Verification items for the finished model (mm, model axes). Face numbers are marked on the shaded views. A direction names the side the tool comes from. Round coordinates to 2 decimals unless told otherwise and drop trailing zeros. Order: outer loops, then holes, each group sorted by start corner. A loop starts at its lowest first (then second) coordinate and runs counter-clockwise, first axis right, second up. Notation, with made-up numbers: M -20.5,-27 L -6.5,-27 A22 ccw -6.5,-2 Z; hole C -12.75,5.5 d10. An arc over 180 degrees is marked long. Write item = value, one per line. Start each with the question number.
from build123d import *

# Parameters (mm, degrees)
CROQUIS1_W              = 20
CROQUIS1_H              = 20
SALIENTE_EXTRUIR1_DEPTH = 30
CROQUIS3_R              = 6.35
CORTAR_EXTRUIR1_DEPTH   = 18
CORTAR_EXTRUIR2_REACH   = 43.231
CROQUIS4_R              = 2
CROQUIS7_W              = 20
CROQUIS7_H              = 20
CROQUIS7_R              = 2
SALIENTE_EXTRUIR3_DEPTH = 1.6
CORTAR_EXTRUIR3_REACH   = 43.231
REDONDEO1_R             = 8


with BuildPart() as part:
    # Croquis1 → Saliente-Extruir1 (new body)
    with BuildSketch(Plane(origin=(0, 0, 0), x_dir=(1, 0, 0), z_dir=(0, 1, 0))):
        with Locations((-10, -10)):
            Rectangle(CROQUIS1_W, CROQUIS1_H)
    extrude(amount=SALIENTE_EXTRUIR1_DEPTH)

    # Croquis3 → Cortar-Extruir1 (cut)
    with BuildSketch(Plane.XY.offset(20)):
        with Locations((-10, 13.75)):
            Circle(CROQUIS3_R)
    extrude(amount=-CORTAR_EXTRUIR1_DEPTH, mode=Mode.SUBTRACT)

    # Cortar-Extruir2: up to this face of the body (flat: up to its plane)
    cortar_extruir2_end = Plane(part.part.faces().sort_by_distance((-10, 0, 10))[0])
    # Croquis4 → Cortar-Extruir2 (cut, up to the picked face)
    with BuildSketch(Plane(origin=(0, 30, 0), x_dir=(1, 0, 0), z_dir=(0, 1, 0)), mode=Mode.PRIVATE) as cortar_extruir2_sk1:
        with Locations(Location((-10, -10, 0), (0, 0, 270))):
            Circle(CROQUIS4_R)
    cortar_extruir2_tool1 = split(extrude(cortar_extruir2_sk1.sketch, amount=-CORTAR_EXTRUIR2_REACH, mode=Mode.PRIVATE), bisect_by=cortar_extruir2_end, keep=Keep.BOTH, mode=Mode.PRIVATE)
    add(cortar_extruir2_tool1.solids().sort_by(Axis((-10, 30, 10), (0, -1, 0)))[0], mode=Mode.SUBTRACT)

    # Croquis7 → Saliente-Extruir3 (add)
    with BuildSketch(Plane.XZ):
        with Locations((-10, 10)):
            Rectangle(CROQUIS7_W, CROQUIS7_H)
        with Locations(Location((-10, 10, 0), (0, 0, 90))):
            Circle(CROQUIS7_R, mode=Mode.SUBTRACT)
    extrude(amount=SALIENTE_EXTRUIR3_DEPTH)

    # Croquis8 → Cortar-Extruir3 (cut, up to next)
    with BuildSketch(Plane.XY.offset(20), mode=Mode.PRIVATE) as cortar_extruir3_sk1:
        with BuildLine():
            Line((-17, 7.75), (-17, 1.4))
            Line((-17, 1.4), (-3, 1.4))
            Line((-3, 1.4), (-3, 7.75))
            Line((-3, 7.75), (-3, 20.65))
            ThreePointArc((-3, 20.65), (-10, 27), (-17, 20.65))
            Line((-17, 20.65), (-17, 7.75))
        make_face()
    cortar_extruir3_tool1 = extrude(cortar_extruir3_sk1.sketch, amount=-CORTAR_EXTRUIR3_REACH, mode=Mode.PRIVATE) & part.part
    add(cortar_extruir3_tool1.solids().sort_by_distance((-10, 13.506159, 20))[0], mode=Mode.SUBTRACT)

    # Redondeo1
    # the kernel refuses this fillet: 8 mm, written as the material it takes off along each edge
    with BuildSketch(Plane(origin=(-20, -21.6, 0), x_dir=(1, 0, 0), z_dir=(0, 1, 0)), Plane(origin=(0, 50, 0), x_dir=(-1, 0, 0), z_dir=(0, -1, 0)), Plane(origin=(-20, -21.6, 20), x_dir=(0, 0, -1), z_dir=(0, 1, 0)), Plane(origin=(0, 50, 20), x_dir=(0, 0, -1), z_dir=(0, -1, 0))) as redondeo1_piece_1:
        with BuildLine():
            CenterArc((REDONDEO1_R, -REDONDEO1_R), REDONDEO1_R, 90, 90)
            Line((0, -REDONDEO1_R), (0, 0))
            Line((0, 0), (REDONDEO1_R, 0))
        make_face()
    extrude(amount=71.6, mode=Mode.SUBTRACT)


solid = part.part
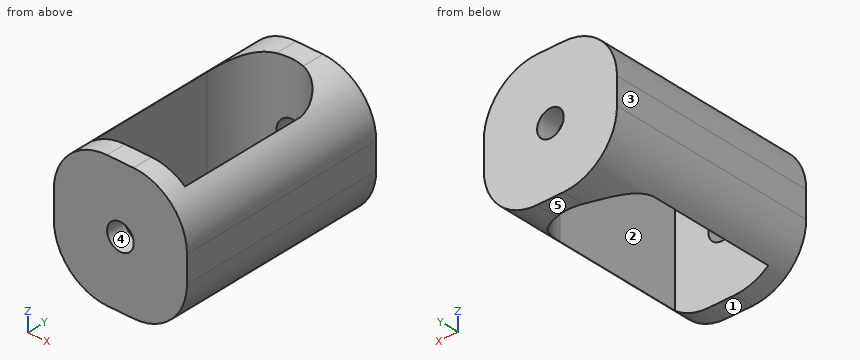
1) Scan lines: probe 1 along X at (y, z) = (27.8, 10); probe 2 along Z at (x, y) = (-10, -0.1); probe 3 along X at (y, z) = (16.5, 9.5). Record each from-to range of solid material in increasing order.
2) Cross-section at A-A, the plane x = -10. Enter the section's corners in (y, z), then the cut area to 3 significant figures.
3) Cross-section at D-D, the plane x = -13.5. Enter the section's corners in (y, z).
4) Cross-section at C-C, the plane z = 10. Enter the section's corners in (x, y), then the cut area to 3 significant figures.
5) Access from +Z, -Z, +X, -X, +Y, -Y to the whole of each face (thin tool, end or side, straight path). Record for the marked faces 1 and 2.
6) Release check for a two-part mould opening along Z. For the marked faces 3, 4 and 5 record: pulls with the +Z half, pulls with the -Z half, needs draft (parallel to the pull), parting line crosses it, or undercut.
7) Gauge pin test, flat ends, axial feed: P1, Ø3.5, axis at x = -10, z = 10, coming from the -Y side; P2, Ø6, axis at y = 10.5, z = 3.5, coming from the +X side. Record the tip position at first contact, or that the pin passes through.
8) Cross-section at B-B, the plane y = 4. Enter the section's corners in (x, z) (3 decimals).
Geometry results:
q1.probe_1 = -20 to -12, -8 to 0
q1.probe_2 = 0 to 8, 12 to 20
q1.probe_3 = -20 to -17, -3 to 0
q2.outline = M -1.6,0 L 1.4,0 L 1.4,8 L -1.6,8 Z; M -1.6,12 L 1.4,12 L 1.4,20 L -1.6,20 Z; M 27,0 L 30,0 L 30,8 L 27,8 Z; M 27,12 L 30,12 L 30,20 L 27,20 Z
q2.area = 96.0 mm^2
q3.outline = M -1.6,0.14 L 1.4,0.14 L 1.4,19.86 L -1.6,19.86 Z; M 26.07,0.14 L 30,0.14 L 30,19.86 L 26.07,19.86 Z
q4.outline = M -20,-1.6 L -12,-1.6 L -12,1.4 L -17,1.4 L -17,20.65 A7.03 cw -12,26.71 L -12,30 L -20,30 Z; M -8,-1.6 L 0,-1.6 L 0,30 L -8,30 L -8,26.71 A7.03 cw -3,20.65 L -3,1.4 L -8,1.4 Z
q4.area = 270 mm^2
q5.face_1 = -Z, +X, -X, +Y, -Y
q5.face_2 = +Z, -Z
q6.face_3 = needs draft
q6.face_4 = undercut
q6.face_5 = pulls with the -Z half
q7.P1 = through
q7.P2 = -0.14
q8.outline = M -20,8 A8 ccw -17,1.755 L -17,18.245 A8 ccw -20,12 Z; M -3,1.755 A8 ccw 0,8 L 0,12 A8 ccw -3,18.245 Z
